```python
from build123d import *

# Parameters (mm, degrees)
SKETCH1_R           = 95
BOSS_EXTRUDE1_DEPTH = 1.7
FILLET1_R           = 1
SKETCH2_R           = 70
BOSS_EXTRUDE2_DEPTH = 18.5
DRAFT3_ANGLE        = -2


with BuildPart() as part:
    # Sketch1 → Boss-Extrude1 (new body)
    with BuildSketch(Plane(origin=(0, 0, 0), x_dir=(1, 0, 0), z_dir=(0, 1, 0))):
        with Locations(Location((0, 0, 0), (0, 0, 270))):
            Circle(SKETCH1_R)
    extrude(amount=BOSS_EXTRUDE1_DEPTH)

    # Fillet1
    fillet1_edges = [part.edges().sort_by_distance(p)[0] for p in [
        (0, 1.7, -95),
    ]]
    fillet(fillet1_edges, radius=FILLET1_R)

    # Sketch2 → Boss-Extrude2 (add)
    with BuildSketch(Plane.XZ):
        with Locations(Location((0, 0, 0), (0, 0, 270))):
            Circle(SKETCH2_R)
    extrude(amount=BOSS_EXTRUDE2_DEPTH)

    # Draft3
    draft3_faces = [part.faces().sort_by_distance(p)[0] for p in [
        (0, -9.25, 70),
    ]]
    draft(draft3_faces, Plane(origin=(0, -18.5, 0), x_dir=(0, 0, -1), z_dir=(0, -1, 0)), DRAFT3_ANGLE)


solid = part.part
```
CAD build for the part. Positions are in the model's coordinates, mm. A direction names the side the tool comes from. Round coordinates to 2 decimals unless told otherwise and drop trailing zeros. Write each loop counter-clockwise with the first axis right and the second up, starting at its lowest first coordinate (ties: lowest second). Pieces come first, ordered by that corner, then holes. Notation, with made-up numbers: (-24, -40) -> (34, -40) arc R37 cw to (34, -4) -> close; hole circle Ø11 at (66, -23.75). An arc over 180 degrees is marked (long way). Answer in a Markdown table with one row per item. Add a question column.
Item 1: Drill centre lines: line 1 (Y direction, x = 29, z = 67.5); line 2 (Z direction, x = 34.5, y = -6.75); line 3 (X direction, y = -15.75, z = 48.5). Where is each one in solid material? Low to high. Write a range as from..to.
Item 2: Saw through at B-B, the plane z = 0. Write the cut outline in (x, y), then the cut area to 3 significant figures.
Item 3: Drop flat-ended pins along their axis: pin 1 Ø8 at (x, y) = (27, -14.5) entering from -Z; pin 2 Ø10 at (x, y) = (55, -11.5) entering from -Z; pin 3 Ø2 at (x, z) = (-58, -47) entering from -Y. Give the stop position or say it passes through.
Item 4: Saw through at A-A, the plane x = 0. Write the cut outline in (y, z).
Item 5: Saw through at C-C, the plane y = -8. Write the cut outline in (x, z), then the cut area to 3 significant figures.
Item 6: Which spindle directions (+Z, -Z, +X, -X, +Y, -Y) get a long thin tool onto all of the face, cutting with end or side? Do faces 1 (the face through (-42.351, -7.065, 55.233)), 2 (the face through (1, 1.7, -1)). Say none if no direction does.
Findings below:
| question | item | result |
|---|---|---|
| 1 | line 1 | y = 0..1.7 |
| 1 | line 2 | z = -60.44..60.44 |
| 1 | line 3 | x = -50.34..50.34 |
| 2 | outline | (-95, 0) -> (-69.35, 0) -> (-70, -18.5) -> (70, -18.5) -> (69.35, 0) -> (95, 0) -> (95, 0.7) arc R1 ccw to (94, 1.7) -> (-94, 1.7) arc R1 ccw to (-95, 0.7) -> close |
| 2 | area | 2,900 mm^2 |
| 3 | pin 1 | stops at z = -65.97 |
| 3 | pin 2 | stops at z = -48.65 |
| 3 | pin 3 | stops at y = 0 |
| 4 | outline | (-18.5, -70) -> (0, -69.35) -> (0, -95) -> (0.7, -95) arc R1 ccw to (1.7, -94) -> (1.7, 94) arc R1 ccw to (0.7, 95) -> (0, 95) -> (0, 69.35) -> (-18.5, 70) -> close |
| 5 | outline | circle Ø139.27 at (0, 0) |
| 5 | area | 15,200 mm^2 |
| 6 | face 1 | none |
| 6 | face 2 | +Z, -Z, +X, -X, +Y |
